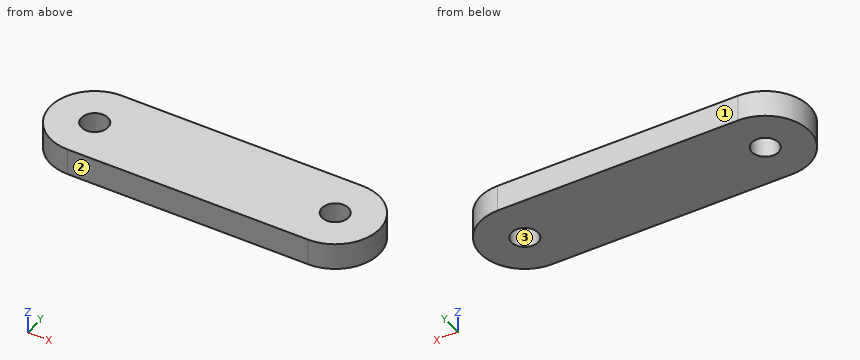
```python
from build123d import *

# Parameters (mm, degrees)
SKETCH_1_R      = 0.75
EXTRUDE_1_DEPTH = 0.75


with BuildPart() as part:
    # 草圖1 → 填料-伸長1 (new body, symmetric)
    with BuildSketch(Plane.XY):
        with BuildLine():
            Line((-6.81, 2.5), (6.81, 2.5))
            ThreePointArc((6.81, 2.5), (9.31, 0), (6.81, -2.5))
            Line((6.81, -2.5), (-6.81, -2.5))
            ThreePointArc((-6.81, -2.5), (-9.31, 0), (-6.81, 2.5))
        make_face()
        with Locations((-6.81, 0)):
            Circle(SKETCH_1_R, mode=Mode.SUBTRACT)
        with Locations((6.81, 0)):
            Circle(SKETCH_1_R, mode=Mode.SUBTRACT)
    extrude(amount=EXTRUDE_1_DEPTH, both=True)


solid = part.part
```
The listing builds one solid part. Answer for the finished solid, in the listing's coordinates (mm). Face numbers are marked on the shaded views. Coordinates: 2 decimals unless noted, no trailing zeros. Loops run counter-clockwise (first coordinate to the right, second up) from the corner with the lowest first, then second, coordinate; pieces in that order, holes last. Notation, with made-up numbers: (-23, 48) - (5, 48) arc R20 cw to (5, 61) - close; hole circle Ø7 at (86.25, 20.25). An arc over 180 degrees is marked (long way). Write item = value, one per line.
1) Section C-C (x = 6.5) is taken. Determine the outline of the cut face in (y, z).
Responses:
outline = (-2.5, -0.75) - (-0.68, -0.75) - (-0.68, 0.75) - (-2.5, 0.75) - close; (0.68, -0.75) - (2.5, -0.75) - (2.5, 0.75) - (0.68, 0.75) - close
2) Find the intervals of material crossed by line 1 along Y through (x, z) = (-6.81, -0.2); line 2 along X through (y, z) = (0.6, -0.3); line 3 along X through (y, z) = (2.2, 0.15), in increasing order.
Responses:
line_1 = -2.5 to -0.75, 0.75 to 2.5
line_2 = -9.24 to -7.26, -6.36 to 6.36, 7.26 to 9.24
line_3 = -8 to 8
3) Section B-B (z = -0.5) is taken. Determine the outline of the cut face in (x, y).
Responses:
outline = (-6.81, -2.5) - (6.81, -2.5) arc R2.5 ccw to (6.81, 2.5) - (-6.81, 2.5) arc R2.5 ccw to start; hole circle Ø1.5 at (-6.81, 0); hole circle Ø1.5 at (6.81, 0)
4) Section D-D (y = 1.1) is taken. Determine the outline of the cut face in (x, z) (3 decimals).
Responses:
outline = (-9.055, -0.75) - (9.055, -0.75) - (9.055, 0.75) - (-9.055, 0.75) - close
5) Section A-A (y = 0) is taken. Determine the outline of the cut face in (x, z).
Responses:
outline = (-9.31, -0.75) - (-7.56, -0.75) - (-7.56, 0.75) - (-9.31, 0.75) - close; (-6.06, -0.75) - (6.06, -0.75) - (6.06, 0.75) - (-6.06, 0.75) - close; (7.56, -0.75) - (9.31, -0.75) - (9.31, 0.75) - (7.56, 0.75) - close
6) Determine the mould class of the marked faces 1, 2 and 3 for opening direction Y: pulls with the +Y half, pulls with the -Y half, needs draft (parallel to the pull), parting line crosses it, or undercut.
Responses:
face_1 = pulls with the +Y half
face_2 = pulls with the -Y half
face_3 = undercut
